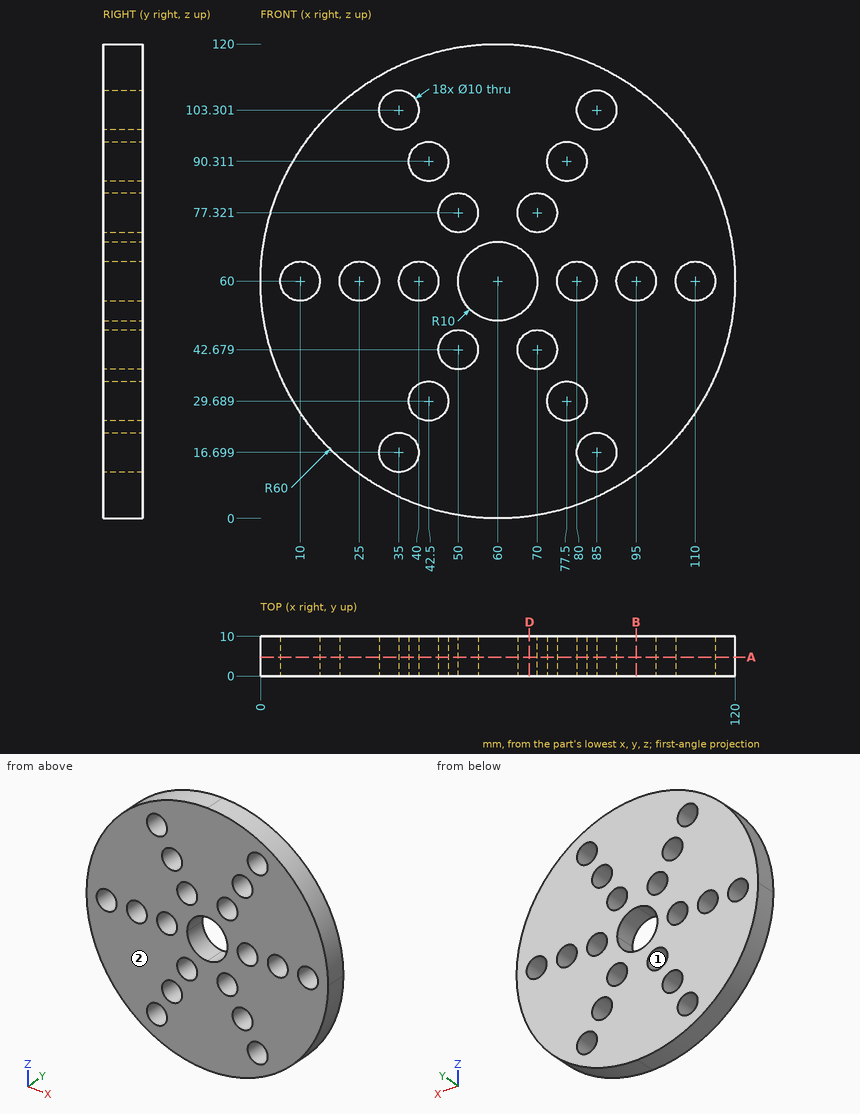
Could you check a few things on this drawing? It's one solid part, dimensions in mm from its lowest x, y, z. Coordinates: 2 decimals unless noted, no trailing zeros. Write each loop counter-clockwise with the first axis right and the second up, starting at its lowest first coordinate (ties: lowest second). Pieces come first, ordered by that corner, then holes. Notation, with made-up numbers: M 0.5,81.25 L 19.5,81.25 A13 cw 19.5,96.25 Z; hole C 27.25,13.25 d3. An arc over 180 degrees is marked long. Answer as CSV lines item,"result". Start each with the question number.
Q1. Will these pins go through, and if not, where does the flat tip stop? pin 1 Ø2 at (x, y) = (101.5, 8) entering from +Z; pin 2 Ø5 at (y, z) = (1, 98.5) entering from +X; pin 3 Ø1.5 at (y, z) = (8.5, 61) entering from -X.
Q2. Suppose I cut it at B-B, the plane x = 95. List the corners of the cut face in (y, z) for me.
Q3. If we mould it in two halves opening along Z, with no side actions, what happens to the marked faces 1 and 2? For each: pulls with the +Z half, pulls with the -Z half, needs draft (parallel to the pull), parting line crosses it, or undercut.
Q4. I need wall thicknesses on probe 1 along X at (y, z) = (7, 28.5) (1 decimal); probe 2 along Z at (x, y) = (68, 8) (1 decimal); probe 3 along X at (y, z) = (1.5, 88.5). Which ranges of each line are inside material? Lowest first, please. Write a range as [from, to].
Q5. Suppose I cut it at A-A, the plane y = 4.75. State how many separate pieces and enclosed holes the cut face has, then the cut area to 3 significant figures.
Q6. Suppose I cut it at D-D, the plane x = 68. List the corners of the cut face in (y, z) for me (1 decimal).
Entries:
1,pin 1,"stops at z = 104.27"
1,pin 2,"stops at x = 108"
1,pin 3,"stops at x = 0"
2,outline,"M 0,11.27 L 10,11.27 L 10,55 L 0,55 Z; M 0,65 L 10,65 L 10,108.73 L 0,108.73 Z"
3,face 1,"undercut"
3,face 2,"needs draft"
4,probe 1,"x = [8.9, 37.6], [47.4, 72.6], [82.4, 111.1]"
4,probe 2,"z = [0.5, 38.1], [47.3, 54], [66, 72.7], [81.9, 119.5]"
4,probe 3,"x = [7.2, 37.84], [47.16, 72.84], [82.16, 112.8]"
5,separate pieces,"1"
5,enclosed holes,"19"
5,area,"9,580 mm²"
6,outline,"M 0,0.5 L 10,0.5 L 10,38.1 L 0,38.1 Z; M 0,47.3 L 10,47.3 L 10,54 L 0,54 Z; M 0,66 L 10,66 L 10,72.7 L 0,72.7 Z; M 0,81.9 L 10,81.9 L 10,119.5 L 0,119.5 Z"
